```python
from build123d import *

# Parameters (mm, degrees)
BOSS_EXTRUDE1_DEPTH = 0.5


with BuildPart() as part:
    # Sketch1 → Boss-Extrude1 (new body)
    with BuildSketch(Plane(origin=(0, 0, 0), x_dir=(-1, 0, 0), z_dir=(0, 0, -1))):
        with BuildLine():
            Line((105, 150), (10, 150))
            ThreePointArc((10, 150), (0, 140), (-10, 150))
            Line((-10, 150), (-105, 150))
            ThreePointArc((-105, 150), (-107.928932188, 142.928932188), (-115, 140))
            Line((-115, 140), (-115, 10))
            ThreePointArc((-115, 10), (-105, 0), (-115, -10))
            Line((-115, -10), (-115, -140))
            ThreePointArc((-115, -140), (-107.928932188, -142.928932188), (-105, -150))
            Line((-105, -150), (-10, -150))
            ThreePointArc((-10, -150), (0, -140), (10, -150))
            Line((10, -150), (105, -150))
            ThreePointArc((105, -150), (107.928932188, -142.928932188), (115, -140))
            Line((115, -140), (115, -10))
            ThreePointArc((115, -10), (105, 0), (115, 10))
            Line((115, 10), (115, 140))
            ThreePointArc((115, 140), (107.928932188, 142.928932188), (105, 150))
        make_face()
        with BuildLine():
            Line((9.5, -94.448385239), (9.5, -90.141798169))
            ThreePointArc((9.5, -90.141798169), (10, -85.192308426), (10.5, -90.141798169))
            Line((10.5, -90.141798169), (10.5, -94.448385239))
            Line((10.5, -94.448385239), (9.5, -94.448385239))
        make_face(mode=Mode.SUBTRACT)
        with BuildLine():
            Line((-10.5, -94.448385239), (-10.5, -90.141798169))
            ThreePointArc((-10.5, -90.141798169), (-10, -85.192308426), (-9.5, -90.141798169))
            Line((-9.5, -90.141798169), (-9.5, -94.448385239))
            Line((-9.5, -94.448385239), (-10.5, -94.448385239))
        make_face(mode=Mode.SUBTRACT)
    extrude(amount=-BOSS_EXTRUDE1_DEPTH)


solid = part.part
```
Check sheet for the modelled part. Datum: model origin and axes. Units: mm. Give positions to 0.01 mm unless a question says otherwise; leave off trailing zeros. Order: outer loops, then holes, each group sorted by start corner. A loop starts at its lowest first (then second) coordinate and runs counter-clockwise, first axis right, second up. Notation, with made-up numbers: M 43,32 L 69,32 A32 cw 69,69 Z; hole C 61.5,12 d7. An arc over 180 degrees is marked long. Answer in a Markdown table with one row per item.
1) Cross-section at B-B, the plane x = 0. Enter the section's corners in (y, z).
Filled sheet:
| item | result |
|---|---|
| outline | M -140,0 L 140,0 L 140,0.5 L -140,0.5 Z |
2) Cross-section at A-A, the plane y = 0. Enter the section's corners in (x, z).
Filled sheet:
| item | result |
|---|---|
| outline | M -105,0 L 105,0 L 105,0.5 L -105,0.5 Z |
3) Gauge pin test, flat end, axial feed: P1, Ø6, axis at x = -10, y = -87.69, coming from the -Z side. Record the tip position at first contact, or that the pin passes through.
Filled sheet:
| item | result |
|---|---|
| P1 | stops at z = 0 |
4) Release check for a two-part mould opening along X. For faces 1 (the cylindrical face through (-0.2, 140, 0.2)), 2 (the cylindrical face through (-108.01, 142.85, 0.25)), 3 (the cylindrical face through (107.85, 143.01, 0.25)), 4 (the cylindrical face through (0.2, -140, 0.2)) record: +X half, -X half, draft (parallel to the pull), parting line (faces both ways), or undercut.
Filled sheet:
| item | result |
|---|---|
| face 1 | undercut |
| face 2 | -X half |
| face 3 | +X half |
| face 4 | undercut |
